```python
from build123d import *

# Parameters (mm, degrees)
AUFSATZ_LINEAR_AUSTRAGEN1_DEPTH = 16


with BuildPart() as part:
    # Skizze1 → Aufsatz-Linear austragen1 (new body)
    with BuildSketch(Plane(origin=(0, 0, 0), x_dir=(1, 0, 0), z_dir=(0, 1, 0))):
        with BuildLine():
            Line((0, 0), (2100, 0))
            Line((2100, 0), (2100, -550))
            Line((2100, -550), (600, -550))
            ThreePointArc((600, -550), (458.578643763, -608.578643763), (400, -750))
            Line((400, -750), (400, -1050))
            Line((400, -1050), (0, -1050))
            Line((0, -1050), (0, 0))
        make_face()
    extrude(amount=AUFSATZ_LINEAR_AUSTRAGEN1_DEPTH)


solid = part.part
```
Geometry check sheet. Reference: the model listing, model coordinates, mm. Give positions to 0.01 mm unless a question says otherwise; leave off trailing zeros. Order: outer loops, then holes, each group sorted by start corner. A loop starts at its lowest first (then second) coordinate and runs counter-clockwise, first axis right, second up. Notation, with made-up numbers: (14.25, 54) - (53.25, 54) arc R34 cw to (53.25, 84) - close; hole circle Ø10 at (1.5, -36.5). An arc over 180 degrees is marked (long way). Write item = value, one per line. Start each with the question number.
1) Gauge pin test, flat ends, axial feed: pin 1 Ø4 at (y, z) = (13.5, 666.5) entering from +X; pin 2 Ø8 at (y, z) = (3, 247.5) entering from -X; pin 3 Ø1 at (x, y) = (1852, 8.5) entering from +Z. Record the tip position at first contact, or that the pin passes through.
2) Section check C-C (z = 656). Enter the section's corners in (x, y), then the cut area to 3 significant figures.
3) Section check A-A (y = 6.5). Enter the section's corners in (x, z), then the cut area to 3 significant figures.
4) Scan lines: L1, parallel to Z at x = 863, y = 13.25; L2, parallel to X at y = 6, z = 890.5; L3, parallel to X at y = 5.75, z = 615. Record each from-to range of solid material in increasing order.
5) Section check B-B (x = 1802). Enter the section's corners in (y, z).
Geometry check:
q1.pin_1 = 419.2
q1.pin_2 = 0
q1.pin_3 = 550
q2.outline = (0, 0) - (423.47, 0) - (423.47, 16) - (0, 16) - close
q2.area = 6,780 mm2
q3.outline = (0, 0) - (2100, 0) - (2100, 550) - (600, 550) arc R200 cw to (400, 750) - (400, 1050) - (0, 1050) - close
q3.area = 1,360,000 mm2
q4.L1 = 0 to 550
q4.L2 = 0 to 400
q4.L3 = 0 to 452.44
q5.outline = (0, 0) - (16, 0) - (16, 550) - (0, 550) - close
